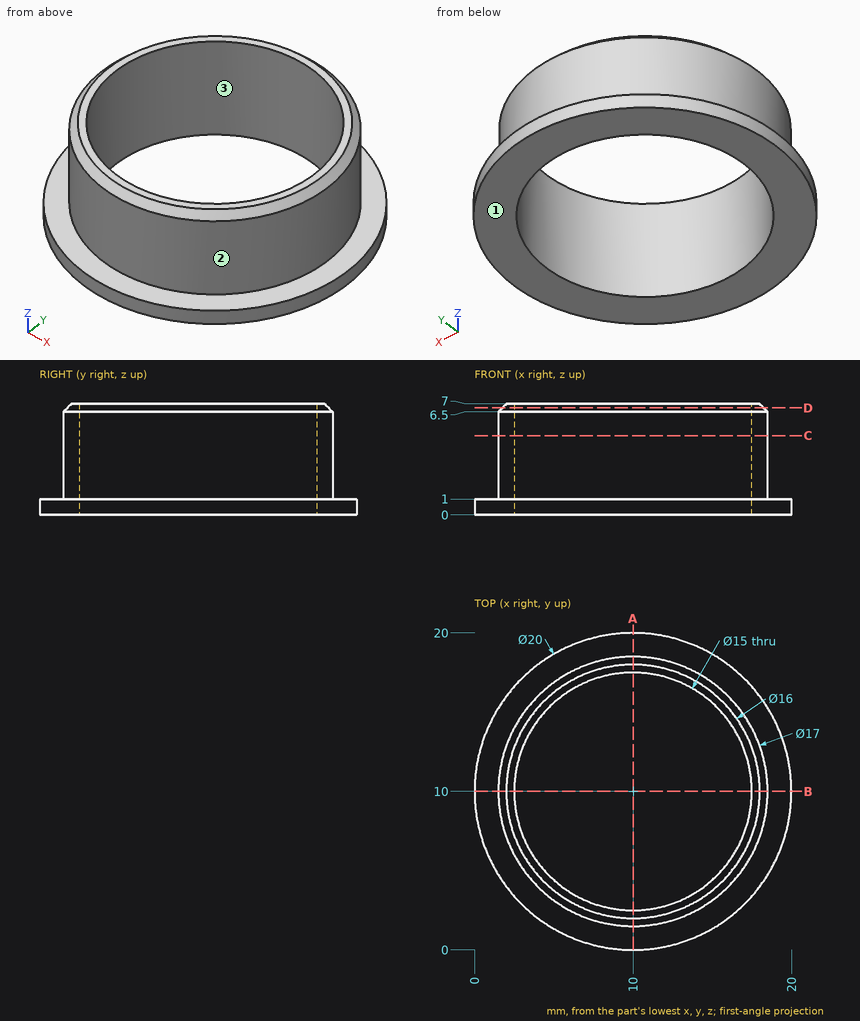
Design review of the part shown in the three views and the two pictorial views. Dimensions are in mm from the part's minimum x, y and z. Give positions to 0.01 mm unless a question says otherwise; leave off trailing zeros. Write each loop counter-clockwise with the first axis right and the second up, starting at its lowest first coordinate (ties: lowest second). Pieces come first, ordered by that corner, then holes. Notation, with made-up numbers: (68, -33.75) - (116, -33.75) arc R18 ccw to (116, -0.75) - close; hole circle Ø8 at (-39, 56). An arc over 180 degrees is marked (long way). Return JSON: item names as keys, results as strings. Group by question number.
(1) We need section A-A, the plane x = 10. Give the boundary of the cut face in (y, z), then the cut area to 4 significant figures.
(2) We need section D-D, the plane z = 6.75. Give the boundary of the cut face in (x, y).
(3) Insertion check: pin 1 (2 mm diameter, centred on y = 13, z = 3.5, fed in from -X); pin 2 (9 mm diameter, centred on x = 10, y = 10, fed in from -Z); pin 3 (3 mm diameter, centred on x = 12.5, z = 6, fed in from -Y). Each pin has a flat end and moves straight along its axis. Give the tip position at first contact, or say it passes through.
(4) To check wall thickness, follow probe 1 along Y at (x, z) = (10, 3.5); probe 2 along X at (y, z) = (16, 1.5); probe 3 along Z at (x, y) = (3.5, 16.25). State the ranges of each line that lie inside material, in increasing order.
(5) Mouldability with a two-part tool opening along Y and no side actions: class the marked faces 1, 2 and 3 as +Y half, -Y half, draft (parallel to the pull), parting line (faces both ways), or undercut.
(6) We need section C-C, the plane z = 5. Give the boundary of the cut face in (x, y).
Reported:
{
 "1": {"outline": "(0, 0) - (2.5, 0) - (2.5, 7) - (2, 7) - (1.5, 6.5) - (1.5, 1) - (0, 1) - close; (17.5, 0) - (20, 0) - (20, 1) - (18.5, 1) - (18.5, 6.5) - (18, 7) - (17.5, 7) - close", "area": "16.75 mm2"},
 "2": {"outline": "circle Ø16.5 at (10, 10); hole circle Ø15 at (10, 10)"},
 "3": {"pin 1": "stops at x = 1.74", "pin 2": "passes through", "pin 3": "stops at y = 1.56"},
 "4": {"probe 1": "y = 1.5 to 2.5, 17.5 to 18.5", "probe 2": "x = 3.98 to 5.5, 14.5 to 16.02", "probe 3": "z = 0 to 1"},
 "5": {"face 1": "draft", "face 2": "parting line", "face 3": "undercut"},
 "6": {"outline": "circle Ø17 at (10, 10); hole circle Ø15 at (10, 10)"}
}
